```python
from build123d import *

# Parameters (mm, degrees)
F0_R     = 15
F0_R_2   = 12
F1_DEPTH = 20
F2_R     = 13
F2_R_2   = 12
F3_DEPTH = 60
F5_DEPTH = 5
F7_DEPTH = 25


with BuildPart() as f1:
    # F0 (on Top) → F1 (new body)
    with BuildSketch(Plane.XY):
        Circle(F0_R)
        Circle(F0_R_2, mode=Mode.SUBTRACT)
    extrude(amount=F1_DEPTH)

    # F2 (on face) → F3 (join)
    with BuildSketch(Plane.XY.offset(20)):
        Circle(F2_R)
        Circle(F2_R_2, mode=Mode.SUBTRACT)
    extrude(amount=F3_DEPTH)

    # F4 (on Top) → F5 (join)
    with BuildSketch(Plane.XY):
        with BuildLine():
            Line((25, 0), (15, 0))
            ThreePointArc((15, 0), (14.9474578418, -1.2543939042), (14.7901994577, -2.5))
            Line((14.7901994577, -2.5), (25, -2.5))
            Line((25, -2.5), (25, 0))
        make_face()
        with BuildLine():
            ThreePointArc((14.7901994577, 2.5), (14.9474578418, 1.2543939042), (15, 0))
            Line((15, 0), (25, 0))
            Line((25, 0), (25, 2.5))
            Line((25, 2.5), (14.7901994577, 2.5))
        make_face()
    extrude(amount=F5_DEPTH)

    # F6 (on Right) → F7 (cut)
    with BuildSketch(Plane.YZ):
        with BuildLine():
            ThreePointArc((0, 60), (3.5355339059, 61.4644660941), (5, 65))
            ThreePointArc((5, 65), (-3.5355339059, 68.5355339059), (0, 60))
        make_face()
    extrude(amount=F7_DEPTH, mode=Mode.SUBTRACT)


solid = f1.part
```
CAD build for the part. Positions are in the model's coordinates, mm. A direction names the side the tool comes from. Round coordinates to 2 decimals unless told otherwise and drop trailing zeros. Order: outer loops, then holes, each group sorted by start corner. A loop starts at its lowest first (then second) coordinate and runs counter-clockwise, first axis right, second up.
Q1. Slice it at D-D (z = 10.5). Write the cut outline in (x, y).
Q2. Which spindle directions (+Z, -Z, +X, -X, +Y, -Y) get a long thin tool onto all of the face, cutting with end or side? Do faces 4 (the flat face through (9, -9, 80)), 5 (the cylindrical face through (-10.316, -7.91, 49.58)), 6 (the flat face through (20, -2.5, 2)). Say none if no direction does.
Q3. Two-plate mould, pull along Y, no slides. Class faces 1 (the cylindrical face through (-11.99, 0.53, 39.44)), 2 (the cylindrical face through (-14.985, 0.66, 9.86)), 3 (the flat face through (20, 2.5, 2)): pulls with the +Y half, pulls with the -Y half, needs draft (parallel to the pull), parting line crosses it, or undercut.
Q4. Slice it at B-B (z = 24.5). Write the cut outline in (x, y).
Q5. Slice it at A-A (x = 7). Write the cut outline in (y, z), and give its area (3 significant figures).
Q6. Drop flat-ended pins along their axis: pin 1 (10 mm diameter, centred on x = 11, z = 46, fed in from -Y); pin 2 (8 mm diameter, centred on x = 14, z = 8, fed in from -Y); pin 3 (4 mm diameter, centred on x = -3.5, z = 20.5, fed in from -Y). Give the stop position or say it passes through.
Q7. Slice it at C-C (y = 9). Write the cut outline in (x, z), and give its area (3 significant figures).
Q8. Wall check: L1, parallel to Y at x = 4, z = 28; L2, parallel to Y at x = 10, z = 19; L3, parallel to X at y = -8.25, z = 38. Give the ranges that are in metal, low to high.
Results below:
1. outline: circle Ø30 at (0, 0); hole circle Ø24 at (0, 0)
2. face 4: +Z, +X, -X, +Y, -Y
2. face 5: +Z
2. face 6: +Z, -Z, +X, -Y
3. face 1: undercut
3. face 2: parting line crosses it
3. face 3: pulls with the +Y half
4. outline: circle Ø26 at (0, 0); hole circle Ø24 at (0, 0)
5. outline: (-13.27, 0) - (-9.75, 0) - (-9.75, 80) - (-10.95, 80) - (-10.95, 20) - (-13.27, 20) - close; (9.75, 0) - (13.27, 0) - (13.27, 20) - (10.95, 20) - (10.95, 80) - (9.75, 80) - close
5. area: 286 mm2
6. pin 1: stops at y = -11.53
6. pin 2: stops at y = -11.18
6. pin 3: stops at y = -14.92
7. outline: (-12, 0) - (-7.94, 0) - (-7.94, 80) - (-9.38, 80) - (-9.38, 20) - (-12, 20) - close; (7.94, 0) - (12, 0) - (12, 20) - (9.38, 20) - (9.38, 80) - (7.94, 80) - close
7. area: 336 mm2
8. L1: y = -12.37 to -11.31, 11.31 to 12.37
8. L2: y = -11.18 to -6.63, 6.63 to 11.18
8. L3: x = -10.05 to -8.71, 8.71 to 10.05
